```python
from build123d import *

# Parameters (mm, degrees)
F1_DEPTH = 2032
F2_R     = 22.225
F3_DEPTH = 50.801


with BuildPart() as f1:
    # F0 (on Front) → F1 (new body)
    with BuildSketch(Plane.XZ):
        with BuildLine():
            ThreePointArc((-84.238662, 22.99025), (-82.37879, 18.500122), (-77.888662, 16.64025))
            Line((-77.888662, 16.64025), (-39.788662, 16.64025))
            ThreePointArc((-39.788662, 16.64025), (-35.298534, 18.500122), (-33.438662, 22.99025))
            Line((-33.438662, 22.99025), (-33.438662, 86.49025))
            ThreePointArc((-33.438662, 86.49025), (-35.298534, 90.980378), (-39.788662, 92.84025))
            Line((-39.788662, 92.84025), (-77.888662, 92.84025))
            ThreePointArc((-77.888662, 92.84025), (-82.37879, 90.980378), (-84.238662, 86.49025))
            Line((-84.238662, 86.49025), (-84.238662, 22.99025))
        make_face()
        with BuildLine():
            ThreePointArc((-79.476162, 86.49025), (-79.011194, 87.612782), (-77.888662, 88.07775))
            Line((-77.888662, 88.07775), (-39.788662, 88.07775))
            ThreePointArc((-39.788662, 88.07775), (-38.66613, 87.612782), (-38.201162, 86.49025))
            Line((-38.201162, 86.49025), (-38.201162, 22.99025))
            ThreePointArc((-38.201162, 22.99025), (-38.66613, 21.867718), (-39.788662, 21.40275))
            Line((-39.788662, 21.40275), (-77.888662, 21.40275))
            ThreePointArc((-77.888662, 21.40275), (-79.011194, 21.867718), (-79.476162, 22.99025))
            Line((-79.476162, 22.99025), (-79.476162, 86.49025))
        make_face(mode=Mode.SUBTRACT)
    extrude(amount=F1_DEPTH)

    # F2 (on face) → F3 (cut, through all)
    with BuildSketch(Plane.YZ.offset(-33.438662)):
        with Locations((-1016, 54.74025)):
            Circle(F2_R)
    extrude(amount=-F3_DEPTH, mode=Mode.SUBTRACT)


solid = f1.part
```
Build history of the part. All positions in model axes, mm. A direction names the side the tool comes from. Round coordinates to 2 decimals unless told otherwise and drop trailing zeros. Write each loop counter-clockwise with the first axis right and the second up, starting at its lowest first coordinate (ties: lowest second). Pieces come first, ordered by that corner, then holes. Notation, with made-up numbers: (-5.5, -21.75) - (35.5, -21.75) arc R29 ccw to (35.5, 5.25) - close; hole circle Ø4 at (-29, 43). An arc over 180 degrees is marked (long way). Write each question's results on one line, items separated by ' | '. Start each with the question number.
Item 1: Drop a flat-ended pin along its axis: P1, Ø12, axis at x = -72, z = 56, coming from the -Y side. Give the stop position or say it passes through.
Item 2: Which spindle directions (+Z, -Z, +X, -X, +Y, -Y) get a long thin tool onto all of the face, cutting with end or side? Do faces 5 (the face through (-33.439, -1002, 75)), 6 (the face through (-59, -1002, 21.403)). Say none if no direction does.
Item 3: Wall check: L1, parallel to Z at x = -44, y = -670; L2, parallel to X at y = -735.5, z = 29; L3, parallel to Z at x = -80, y = -1016. Give the ranges that are in metal, low to high. Write a range as [from, to].
Item 4: Mould opens along Z. For faces 1 (the face through (-84.239, -1002, 34)), 2 (the face through (-38.201, -1002, 34)), 3 (the face through (-59, -1002, 92.84)), 4 (the face through (-81.824, -1038.204, 55.717)) say: pulls with the +Z half, pulls with the -Z half, needs draft (parallel to the pull), parting line crosses it, or undercut.
Item 5: Saw through at B-B (x = -66). Write the cut outline in (y, z), and give its area (3 significant figures).
Results are:
1) P1: passes through
2) face 5: +Z, -Z, +X, +Y, -Y | face 6: +Y, -Y
3) L1: z = [16.64, 21.4], [88.08, 92.84] | L2: x = [-84.24, -79.48], [-38.2, -33.44] | L3: z = [17, 32.52], [76.97, 92.48]
4) face 1: needs draft | face 2: undercut | face 3: pulls with the +Z half | face 4: undercut
5) outline: (-2032, 16.64) - (0, 16.64) - (0, 21.4) - (-2032, 21.4) - close; (-2032, 88.08) - (0, 88.08) - (0, 92.84) - (-2032, 92.84) - close | area: 19,400 mm²
